Geometry check sheet. Reference: the model listing, model coordinates, mm. A direction names the side the tool comes from. Give positions to 0.01 mm unless a question says otherwise; leave off trailing zeros. Order: outer loops, then holes, each group sorted by start corner. A loop starts at its lowest first (then second) coordinate and runs counter-clockwise, first axis right, second up. Notation, with made-up numbers: M 25.25,74.25 L 77.25,74.25 A21 cw 77.25,92.25 Z; hole C -5.75,5.5 d1. An arc over 180 degrees is marked long. Answer as CSV lines item,"result". Start each with the question number.
Q1. Section check A-A, the plane y = 13. Record the boundary of the cut face in (x, z), then the cut area to 3 significant figures.
Q2. Go/stop test with flat-tipped pins: pin 1 (4 mm diameter, centred on y = 10.5, z = 11, fed in from -X); pin 2 (3 mm diameter, centred on x = -12.5, z = 11, fed in from +Y); pin 3 (4 mm diameter, centred on x = -14.5, y = 14, fed in from +Z). Record where each tip stops, or that it passes through.
Q3. Set-up check for faces 4 (the flat face through (-13, 6, 5)), 5 (the flat face through (-3, 20, 5)): record each of +Z, -Z, +X, -X, +Y, -Y from which the full face is reachable in a straight line by a thin tool's end or side.
Q4. Section check B-B, the plane x = -13. Record the boundary of the cut face in (y, z).
Q5. Section check C-C, the plane z = 8.75. Record the boundary of the cut face in (x, y), then the cut area to 4 significant figures.
Q6. Thickness scan on line 1 (Z direction, x = -1.6, y = 13); line 2 (Y direction, x = -9, z = 14). Record the ranges inside material, lowest first.
Q7. Mould release check, pull along X, two halves, no side actions. Record for faces 1 (the flat face through (-10, 0, 10)), 2 (the flat face through (-5, 6, 13)), 3 (the cylindrical face through (-14.77, 14.62, 1.97)): +X half, -X half, draft (parallel to the pull), parting line (faces both ways), or undercut.
```python
from build123d import *

# Parameters (mm, degrees)
SKETCH001_W     = 20
SKETCH001_H     = 20
SKETCH001_R     = 2.4
PAD001_DEPTH    = 4
SKETCH002_W     = 20
SKETCH002_H     = 20
SKETCH002_R     = 2.4
PAD002_DEPTH    = 4
SKETCH_W        = 20
SKETCH_H        = 20
SKETCH_R        = 2.4
PAD_DEPTH       = 4
CHAMFER_SIZE    = 3
CHAMFER001_SIZE = 3
CHAMFER002_SIZE = 3


with BuildPart() as pad001:
    # Sketch001 → Pad001 (new body)
    with BuildSketch(Plane.XZ.offset(-4)):
        with Locations((-10, 10)):
            Rectangle(SKETCH001_W, SKETCH001_H)
        with Locations((-13, 13)):
            Circle(SKETCH001_R, mode=Mode.SUBTRACT)
    extrude(amount=PAD001_DEPTH)


with BuildPart() as pad002:
    # Sketch002 → Pad002 (new body)
    with BuildSketch(Plane.YZ.offset(-4)):
        with Locations((10, 10)):
            Rectangle(SKETCH002_W, SKETCH002_H)
        with Locations((13, 13)):
            Circle(SKETCH002_R, mode=Mode.SUBTRACT)
    extrude(amount=PAD002_DEPTH)


with BuildPart() as chamfer002:
    # Sketch → Pad (new body)
    with BuildSketch(Plane.XY):
        with Locations((-10, 10)):
            Rectangle(SKETCH_W, SKETCH_H)
        with Locations((-13, 13)):
            Circle(SKETCH_R, mode=Mode.SUBTRACT)
    extrude(amount=PAD_DEPTH)

    # Fusion: union Pad001, Pad002
    add(pad001.part)
    add(pad002.part)

    # Chamfer
    chamfer_edges = [chamfer002.edges().sort_by_distance(p)[0] for p in [
        (-4, 4, 12),
    ]]
    chamfer(chamfer_edges, length=CHAMFER_SIZE)

    # Chamfer001
    chamfer001_edges = [chamfer002.edges().sort_by_distance(p)[0] for p in [
        (-13.5, 4, 4),
    ]]
    chamfer(chamfer001_edges, length=CHAMFER001_SIZE)

    # Chamfer002
    chamfer002_edges = [chamfer002.edges().sort_by_distance(p)[0] for p in [
        (-4, 13.5, 4),
    ]]
    chamfer(chamfer002_edges, length=CHAMFER002_SIZE)


solid = chamfer002.part
```
Answer block:
1,outline,"M -20,0 L -15.4,0 L -15.4,4 L -20,4 Z; M -10.6,0 L 0,0 L 0,10.6 L -4,10.6 L -4,7 L -7,4 L -10.6,4 Z; M -4,15.4 L 0,15.4 L 0,20 L -4,20 Z"
1,area,"110 mm2"
2,pin 1,"stops at x = -4"
2,pin 2,"stops at y = 4"
2,pin 3,"stops at z = 4"
3,face 4,"+Z, -X, +Y"
3,face 5,"+Z, -Z, +X, -X, +Y"
4,outline,"M 0,0 L 10.6,0 L 10.6,4 L 7,4 L 4,7 L 4,10.6 L 0,10.6 Z; M 0,15.4 L 4,15.4 L 4,20 L 0,20 Z; M 15.4,0 L 20,0 L 20,4 L 15.4,4 Z"
5,outline,"M -20,0 L 0,0 L 0,20 L -4,20 L -4,7 L -7,4 L -20,4 Z"
5,area,"148.5 mm2"
6,line 1,"z = 0 to 10.6, 15.4 to 20"
6,line 2,"y = 0 to 4"
7,face 1,"draft"
7,face 2,"-X half"
7,face 3,"undercut"
